```python
from build123d import *

# Parameters (mm, degrees)
SKETCH2_R           = 3.175
SKETCH2_R_2         = 3.96875
BOSS_EXTRUDE1_DEPTH = 6.35
FILLET1_R           = 9.525
FILLET3_R           = 38.1


with BuildPart() as part:
    # Sketch2 → Boss-Extrude1 (new body)
    with BuildSketch(Plane(origin=(0, 0, 0), x_dir=(1, 0, 0), z_dir=(0, 1, 0))):
        with BuildLine():
            ThreePointArc((-148.920700374, 9.525), (-149.225, 0), (-148.920700374, -9.525))
            Line((-148.920700374, -9.525), (-9.525, -9.525))
            Line((-9.525, -9.525), (-9.525, -148.920700374))
            ThreePointArc((-9.525, -148.920700374), (0, -149.225), (9.525, -148.920700374))
            Line((9.525, -148.920700374), (9.525, -9.525))
            Line((9.525, -9.525), (148.920700374, -9.525))
            ThreePointArc((148.920700374, -9.525), (149.148905692, -4.764929781), (149.225, 0))
            ThreePointArc((149.225, 0), (149.148905692, 4.764929781), (148.920700374, 9.525))
            Line((148.920700374, 9.525), (9.525, 9.525))
            Line((9.525, 9.525), (9.525, 148.920700374))
            ThreePointArc((9.525, 148.920700374), (0, 149.225), (-9.525, 148.920700374))
            Line((-9.525, 148.920700374), (-9.525, 9.525))
            Line((-9.525, 9.525), (-148.920700374, 9.525))
        make_face()
        with Locations(Location((-144.4625, 0, 0), (0, 0, 270))):
            Circle(SKETCH2_R, mode=Mode.SUBTRACT)
        with Locations(Location((0, -144.4625, 0), (0, 0, 270))):
            Circle(SKETCH2_R, mode=Mode.SUBTRACT)
        with Locations(Location((144.4625, 0, 0), (0, 0, 270))):
            Circle(SKETCH2_R, mode=Mode.SUBTRACT)
        with Locations(Location((0, 144.4625, 0), (0, 0, 270))):
            Circle(SKETCH2_R, mode=Mode.SUBTRACT)
        with Locations(Location((0, 0, 0), (0, 0, 270))):
            Circle(SKETCH2_R_2, mode=Mode.SUBTRACT)
    extrude(amount=BOSS_EXTRUDE1_DEPTH)

    # Fillet1
    fillet1_edges = [part.edges().sort_by_distance(p)[0] for p in [
        (-9.525, 3.175, -148.920700374),
        (9.525, 3.175, -148.920700374),
        (148.920700374, 3.175, -9.525),
        (148.920700374, 3.175, 9.525),
        (9.525, 3.175, 148.920700374),
        (-9.525, 3.175, 148.920700374),
        (-148.920700374, 3.175, -9.525),
        (-148.920700374, 3.175, 9.525),
    ]]
    fillet(fillet1_edges, radius=FILLET1_R - 0.0001)  # a hair under: the kernel refuses the full size

    # Fillet3
    fillet3_edges = [part.edges().sort_by_distance(p)[0] for p in [
        (9.525, 3.175, 9.525),
        (-9.525, 3.175, 9.525),
        (-9.525, 3.175, -9.525),
        (9.525, 3.175, -9.525),
    ]]
    fillet(fillet3_edges, radius=FILLET3_R)


solid = part.part
```
Input: part model. Units: mm. Frame: model coordinates. A direction names the side the tool comes from. Give positions to 0.01 mm unless a question says otherwise; leave off trailing zeros. Loops run counter-clockwise (first coordinate to the right, second up) from the corner with the lowest first, then second, coordinate; pieces in that order, holes last.
1) Contact query for flat-ended pins moving along their axis: pin 1 (3 mm diameter, centred on x = -41.5, y = 5, fed in from -Z); pin 2 (1.9 mm diameter, centred on y = 3, z = 114, fed in from -X) (3 decimals); pin 3 (1 mm diameter, centred on x = 38, y = 3, fed in from +Z) (3 decimals); pin 4 (5.5 mm diameter, centred on x = 144.46, z = 0, fed in from +Y). Output: stop coordinate, or through.
A:
pin 1: stops at z = -10.3
pin 2: stops at x = -9.525
pin 3: stops at z = 10.895
pin 4: passes through
2) Section query B-B on x = -37.5. Return the cut outline in (y, z), and give its area (3 significant figures).
A:
outline: (0, -10.89) - (6.35, -10.89) - (6.35, 10.89) - (0, 10.89) - close
area: 138 mm2
3) Mould query, pull axis X, two halves, no side actions, for faces 1 (the cylindrical face through (-20.98, 3.22, -20.39)), 2 (the cylindrical face through (141.363, 3.131, -0.688)), 3 (the flat face through (9.525, 3, 94)). Classes: released by +X, released by -X, zero draft, split by the parting line, or undercut.
A:
face 1: released by -X
face 2: undercut
face 3: released by +X
4) Section query A-A on z = 118. Return the cut outline in (x, y) (3 decimals), and give its area (3 significant figures).
A:
outline: (-9.525, 0) - (9.525, 0) - (9.525, 6.35) - (-9.525, 6.35) - close
area: 121 mm2
5) Line query: L1, parallel to X at y = 3.75, z = 0 (1 decimal); L2, parallel to Z at x = -85, y = 1.25 (3 decimals). Output: solid intervals per line, ascending.
A:
L1: x = -149.2 to -147.6, -141.3 to -4, 4 to 141.3, 147.6 to 149.2
L2: z = -9.525 to 9.525
6) Reachability of faces 4 (the cylindrical face through (-1.2, 3.1, 147.4)), 5 (the flat face through (93, 3, 9.525)), 6 (the flat face through (-93, 3, -9.525)), 7 (the flat face through (-94, 3, 9.525)) from +Z, -Z, +X, -X, +Y, -Y: full face, straight path, thin tool, end or side. Return the list, or none.
A:
face 4: +Y, -Y
face 5: +Z, +X, +Y, -Y
face 6: -Z, -X, +Y, -Y
face 7: +Z, -X, +Y, -Y
